```python
from build123d import *

# Parameters (mm, degrees)
BOSS_EXTRUDE1_DEPTH = 0.3
BOSS_EXTRUDE2_DEPTH = 1.3
SKETCH3_W           = 1.05
SKETCH3_H           = 0.7
CUT_EXTRUDE1_DEPTH  = 0.3
FILLET1_R           = 0.2
SKETCH4_OUTSIDE_W   = 16.684
SKETCH4_OUTSIDE_H   = 6.284
CUT_EXTRUDE3_DEPTH  = 1.05
SKETCH5_OUTSIDE_W   = 16.684
SKETCH5_OUTSIDE_H   = 6.284
CUT_EXTRUDE4_DEPTH  = 1.05


with BuildPart() as part:
    # Sketch1 → Boss-Extrude1 (new body)
    with BuildSketch(Plane(origin=(0, 0, 0), x_dir=(1, 0, 0), z_dir=(0, 1, 0))):
        Polygon((-6, 1.85236673), (6, 1.5), (6, -1.5), (-6, -1.84763327), (-6, -0.84763327), (0, -0.5), (0, 0.5), (-6, 0.85236673), align=None)
    extrude(amount=BOSS_EXTRUDE1_DEPTH)

    # Sketch2 → Boss-Extrude2 (add)
    with BuildSketch(Plane(origin=(0, 0.3, 0), x_dir=(1, 0, 0), z_dir=(0, 1, 0))):
        Polygon((-6, 0.85236673), (-6, 2.90236673), (-5.7, 2.90236673), (-5.7, 0.834748394), align=None)
        Polygon((-6, -0.84763327), (-6, -2.89763327), (-5.7, -2.89763327), (-5.7, -0.830251606), align=None)
    extrude(amount=BOSS_EXTRUDE2_DEPTH)

    # Sketch3 → Cut-Extrude1 (cut)
    with BuildSketch(Plane.ZY.offset(6)):
        with Locations((-2.37736673, 0.65)):
            Rectangle(SKETCH3_W, SKETCH3_H)
        with Locations((2.37263327, 0.65)):
            Rectangle(SKETCH3_W, SKETCH3_H)
    extrude(amount=-CUT_EXTRUDE1_DEPTH, mode=Mode.SUBTRACT)

    # Fillet1
    fillet1_edges = [part.edges().sort_by_distance(p)[0] for p in [
        (-6, 0, -1.35236673),
        (-6, 0, 1.34763327),
    ]]
    fillet(fillet1_edges, radius=FILLET1_R)

    # Sketch4 outside → Cut-Extrude3 (cut)
    with BuildSketch(Plane(origin=(0, 0, -2.90236673), x_dir=(-1, 0, 0), z_dir=(0, 0, -1))):
        with Locations((0, 0.8)):
            Rectangle(SKETCH4_OUTSIDE_W, SKETCH4_OUTSIDE_H)
        with BuildLine():
            Line((5.7, 1.559807621), (5.7, 1.040192379))
            ThreePointArc((5.7, 1.040192379), (5.85, 1), (6, 1.040192379))
            Line((6, 1.040192379), (6, 1.559807621))
            ThreePointArc((6, 1.559807621), (5.85, 1.6), (5.7, 1.559807621))
        make_face(mode=Mode.SUBTRACT)
    extrude(amount=-CUT_EXTRUDE3_DEPTH, mode=Mode.SUBTRACT)

    # Sketch5 outside → Cut-Extrude4 (cut)
    with BuildSketch(Plane.XY.offset(2.89763327)):
        with Locations((0, 0.8)):
            Rectangle(SKETCH5_OUTSIDE_W, SKETCH5_OUTSIDE_H)
        with BuildLine():
            Line((-5.7, 1.559807621), (-5.7, 1.040192379))
            ThreePointArc((-5.7, 1.040192379), (-5.85, 1), (-6, 1.040192379))
            Line((-6, 1.040192379), (-6, 1.559807621))
            ThreePointArc((-6, 1.559807621), (-5.85, 1.6), (-5.7, 1.559807621))
        make_face(mode=Mode.SUBTRACT)
    extrude(amount=-CUT_EXTRUDE4_DEPTH, mode=Mode.SUBTRACT)


solid = part.part
```
The listing builds one solid part. Answer for the finished solid, in the listing's coordinates (mm). A direction names the side the tool comes from. Round coordinates to 2 decimals unless told otherwise and drop trailing zeros. Order: outer loops, then holes, each group sorted by start corner. A loop starts at its lowest first (then second) coordinate and runs counter-clockwise, first axis right, second up. Notation, with made-up numbers: (80.25, -15) - (124.25, -15) arc R15 cw to (124.25, 6) - close; hole circle Ø2 at (40, 69.25). An arc over 180 degrees is marked (long way). Put each result on its own line as item: value. Start each with the question number.
(1) Determine the mould class of faces 3 (the flat face through (-6, 1.05, 1.66)), 4 (the flat face through (0.2, 0.3, 0)), 5 (the flat face through (0.2, 0, 0)) for opening direction Y: released by +Y, released by -Y, zero draft, split by the parting line, or undercut.
(2) Straight lines are drawn through the part: probe 1 along Y at (x, z) = (-1.25, -1.45); probe 2 along X at (y, z) = (1, 0.95); probe 3 along Z at (x, y) = (3.5, 0.1). For each, find the intervals that lie inside material, in ascending order. Write a range as from..to.
(3) Given P1, Ø0.6, axis at y = 1.5, z = -2.5, coming from the +X side; P2, Ø3, axis at x = 1.5, z = -0.5, coming from the +Y side, each flat-ended and moving along its own axis, determine where each tip first touches the part or whether it passes through.
(4) Find section D-D (x = 4.75). Give the vertices of the cut face in (y, z).
(5) Find section A-A (y = 0.65). Give the vertices of the cut face in (x, z).
(6) Find section C-C (x = -1). Give the vertices of the cut face in (y, z), plus the area to 4 significant figures.
(7) For faces 1 (the flat face through (-6, 1, -1.6)), 2 (the flat face through (-5.7, 1.1, -1.7)), determine the directions among +Z, -Z, +X, -X, +Y, -Y from which every point of the face is accessible in a straight line to the end or side of a thin tool.
(8) Find section B-B (z = 1.2). Give the vertices of the cut face in (x, y), plus the area to 3 significant figures.
Reply:
1. face 3: zero draft
1. face 4: released by +Y
1. face 5: released by -Y
2. probe 1: 0..0.3
2. probe 2: -6..-5.7
2. probe 3: -1.57..1.57
3. P1: x = -5.7
3. P2: y = 0.3
4. outline: (0, -1.54) - (0.3, -1.54) - (0.3, 1.54) - (0, 1.54) - close
5. outline: (-6, -1.85) - (-5.7, -1.85) - (-5.7, -0.83) - (-6, -0.85) - close; (-6, 0.85) - (-5.7, 0.83) - (-5.7, 1.85) - (-6, 1.85) - close
6. outline: (0, -1.71) - (0.3, -1.71) - (0.3, -0.56) - (0, -0.56) - close; (0, 0.56) - (0.3, 0.56) - (0.3, 1.7) - (0, 1.7) - close
6. area: 0.6875 mm^2
7. face 1: +Z, -Z, -X, +Y, -Y
7. face 2: +Z, -Z, +X, +Y
8. outline: (-6, 0.2) arc R0.2 ccw to (-5.8, 0) - (6, 0) - (6, 0.3) - (-5.7, 0.3) - (-5.7, 1.6) - (-6, 1.6) - close
8. area: 3.98 mm^2
